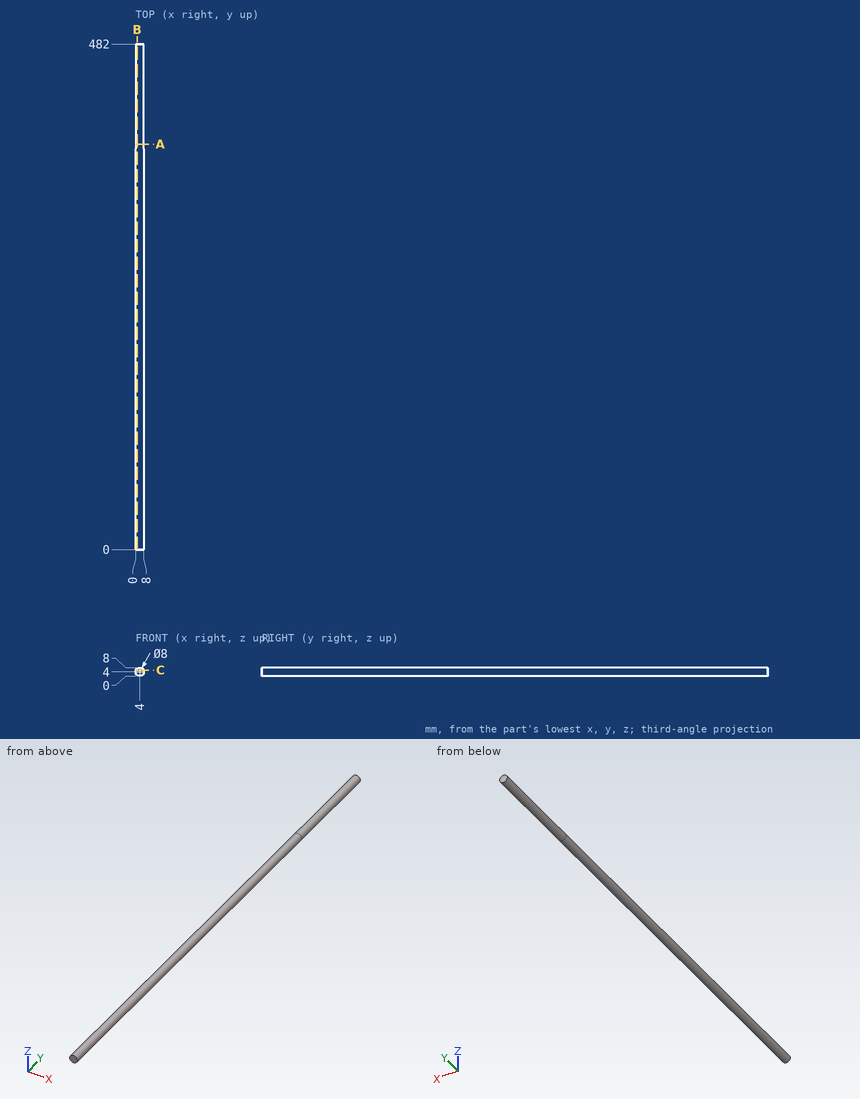
Design review of the part shown in the three views and the two pictorial views. Dimensions are in mm from the part's minimum x, y and z. Coordinates: 2 decimals unless noted, no trailing zeros. Loops run counter-clockwise (first coordinate to the right, second up) from the corner with the lowest first, then second, coordinate; pieces in that order, holes last. Notation, with made-up numbers: M 42,87.5 L 49,87.5 A29 cw 49,122.5 Z; hole C -34.5,54 d11. An arc over 180 degrees is marked long. Put each result on its own line as item: value. Start each with the question number.
Q1. Add section B-B (x = 1.5). Write out the cut boundary in (y, z).
Q2. Wall thickness on line 1 (X direction, y = 350.5, z = 3.25); line 2 (X direction, y = 130, z = 4.5); line 3 (Z direction, x = 6.25, y = 373): over which ranges is each line inside the solid? List them lowest first.
Q3. Add section A-A (y = 386.5). Write out the cut boundary in (x, z), and give its area (3 significant figures).
Q4. Add section C-C (z = 5.5). Write out the cut boundary in (x, y), and give its area (3 significant figures).
Q5. Clearance check with flat-ended pins moving along their axes: pin 1 (4 mm diameter, centred on y = 307, z = 4.5, fed in from -X); pin 2 (1.5 mm diameter, centred on x = 5, y = 55.5, fed in from +Z). State where each tip first meets the part, or that it passes through.
Answers:
1. outline: M 0,0.88 L 482,0.88 L 482,7.12 L 0,7.12 Z
2. line 1: x = 0.07 to 7.93
2. line 2: x = 0.03 to 7.97
2. line 3: z = 0.69 to 7.31
3. outline: C 4,4 d8
3. area: 50.3 mm^2
4. outline: M 0.29,0 L 7.71,0 L 7.71,482 L 0.29,482 Z
4. area: 3,570 mm^2
5. pin 1: stops at x = 0
5. pin 2: stops at z = 7.99
